Input: part model. Units: mm. Frame: model coordinates. A direction names the side the tool comes from. Coordinates: 2 decimals unless noted, no trailing zeros. Loops run counter-clockwise (first coordinate to the right, second up) from the corner with the lowest first, then second, coordinate; pieces in that order, holes last.
```python
from build123d import *

# Parameters (mm, degrees)
F0_R     = 8.5
F1_DEPTH = 14
F2_R     = 11.5
F2_R_2   = 8.5
F4_DEPTH = 2
F5_SIZE  = 1.99999
F3_R     = 11.5
F3_R_2   = 8.5
F6_DEPTH = 2
F7_SIZE  = 1.99999
F8_R     = 7.5
F9_DEPTH = 14.001


# Not quite as in the source:
# - a fillet or chamfer is up to 0.001 mm smaller than in the source, because OpenCascade refuses the exact size


with BuildPart() as f1:
    # F0 (on Top) → F1 (new body)
    with BuildSketch(Plane.XY):
        Circle(F0_R)
    extrude(amount=F1_DEPTH)

    # F2 (on face) → F4 (join)
    with BuildSketch(Plane.XY.offset(14)):
        Circle(F2_R)
        Circle(F2_R_2, mode=Mode.SUBTRACT)
    extrude(amount=-F4_DEPTH)

    # F5 (size 2 in the source; OpenCascade refuses exactly that, so slightly less here)
    f5_edges = [f1.edges().sort_by_distance(p)[0] for p in [
        (-11.5, 0, 12),
    ]]
    chamfer(f5_edges, length=F5_SIZE)

    # F3 (on face) → F6 (join)
    with BuildSketch(Plane(origin=(0, 0, 0), x_dir=(1, 0, 0), z_dir=(0, 0, -1))):
        Circle(F3_R)
        Circle(F3_R_2, mode=Mode.SUBTRACT)
    extrude(amount=-F6_DEPTH)

    # F7 (size 2 in the source; OpenCascade refuses exactly that, so slightly less here)
    f7_edges = [f1.edges().sort_by_distance(p)[0] for p in [
        (-11.5, 0, 2),
    ]]
    chamfer(f7_edges, length=F7_SIZE)

    # F8 (on face) → F9 (cut, through all)
    with BuildSketch(Plane.XY.offset(14)):
        Circle(F8_R)
    extrude(amount=-F9_DEPTH, mode=Mode.SUBTRACT)


solid = f1.part
```
Item 1: Reachability of faces 1 (the face through (-7.493, 0.33, 7.098)), 2 (the face through (4.57, 7.167, 6.93)) from +Z, -Z, +X, -X, +Y, -Y: full face, straight path, thin tool, end or side. Return the list, or none.
Result:
face 1: +Z, -Z
face 2: none
Item 2: Section query C-C (z = 7.75). Output: boundary loops of the cut face in (x, y).
Result:
outline: circle Ø17 at (0, 0); hole circle Ø15 at (0, 0)
Item 3: Section query D-D (z = 1.5). Output: boundary loops of the cut face in (x, y), then the cut area to 3 significant figures.
Result:
outline: circle Ø20 at (0, 0); hole circle Ø15 at (0, 0)
area: 137 mm2
Item 4: Mould query, pull axis Z, two halves, no side actions, for faces 3 (the face through (-2.2, -8.4, 12)), 4 (the face through (8, 0, 0)), 5 (the face through (8, 0, 14)). Classes: +Z half, -Z half, draft (parallel to the pull), parting line (faces both ways), or undercut.
Result:
face 3: undercut
face 4: -Z half
face 5: +Z half
Item 5: Line query: L1, parallel to Y at x = 0, z = 9.5; L2, parallel to Z at x = -1, y = 9; L3, parallel to Z at x = 5.25, y = 9. Output: solid intervals per line, ascending.
Result:
L1: y = -8.5 to -7.5, 7.5 to 8.5
L2: z = 0 to 2, 12 to 14
L3: z = 0 to 1.08, 12.92 to 14
Item 6: Contact query for flat-ended pins moving along their axis: P1, Ø1, axis at y = -7, z = 6, coming from the +X side; P2, Ø2, axis at y = -1.5, z = 7, coming from the -X side; P3, Ø5, axis at y = -8, z = 8, coming from the -X side. Output: stop coordinate, or through.
Result:
P1: stops at x = 5.48
P2: stops at x = -8.49
P3: stops at x = -6.48
